Work out the finished part from the listing and answer in its coordinate system (mm). A direction names the side the tool comes from. Coordinates: 2 decimals unless noted, no trailing zeros. Loops run counter-clockwise (first coordinate to the right, second up) from the corner with the lowest first, then second, coordinate; pieces in that order, holes last. Notation, with made-up numbers: M 87,-9.5 L 136,-9.5 A14 ccw 136,4.5 Z; hole C 87,-4.5 d6. An arc over 180 degrees is marked long. Write each question's results on one line, items separated by ' | '.
```python
from build123d import *

# Parameters (mm, degrees)
F0_W     = 2
F0_H     = 35
F1_DEPTH = 22
F2_R     = 1
F3_DEPTH = 25
F4_W     = 1
F4_H     = 35
F4_W_2   = 2
F5_DEPTH = 2
F8_R     = 4.5
F8_R_2   = 2.5
F9_DEPTH = 8.5


# Not quite as in the source:
# - a feature names something its author has since deleted; it is built from what else it names


with BuildPart() as f1:
    # F0 (on Front) → F1 (new body)
    with BuildSketch(Plane.XZ):
        Rectangle(F0_W, F0_H)
    extrude(amount=F1_DEPTH)

    # F2 (on face) → F3 (cut)
    with BuildSketch(Plane(origin=(-1, 0, 0), x_dir=(0, -1, 0), z_dir=(-1, 0, 0))):
        with Locations((5, 10)):
            Circle(F2_R)
        with Locations((15, 10)):
            Circle(F2_R)
        with Locations((15, 0)):
            Circle(F2_R)
        with Locations((5, 0)):
            Circle(F2_R)
        with Locations((5, -10)):
            Circle(F2_R)
        with Locations((15, -10)):
            Circle(F2_R)
    extrude(amount=-F3_DEPTH, mode=Mode.SUBTRACT)

    # F4 (on face) → F5 (join)
    with BuildSketch(Plane.XZ.offset(22)):
        with Locations((-1.5, 0)):
            Rectangle(F4_W, F4_H)
        with Locations((1.5, 0)):
            Rectangle(F4_W, F4_H)
        Rectangle(F4_W_2, F4_H)
    extrude(amount=F5_DEPTH)

    # F8 (on offset) + F6 (on face) → F9 (join)
    with BuildSketch(Plane(origin=(0, 0, 0), x_dir=(1, 0, 0), z_dir=(0, 0, -1))):
        with Locations((0, 26.5)):
            Circle(F8_R)
        with Locations((0, 26.5)):
            Circle(F8_R_2, mode=Mode.SUBTRACT)
    with BuildSketch(Plane(origin=(0, 0, -17.5), x_dir=(1, 0, 0), z_dir=(0, 0, -1))):
        with BuildLine():
            Line((-2, 24), (0, 24))
            Line((0, 24), (2, 24))
            Line((2, 24), (2, 22.4688711259))
            ThreePointArc((2, 22.4688711259), (3.8242646352, 24.1282917549), (4.5, 26.5))
            ThreePointArc((4.5, 26.5), (-2.3717082451, 30.3242646352), (-2, 22.4688711259))
            Line((-2, 22.4688711259), (-2, 24))
        make_face()
        with BuildLine():
            ThreePointArc((0, 24), (-1.767766953, 28.267766953), (2.5, 26.5))
            ThreePointArc((2.5, 26.5), (1.767766953, 24.732233047), (0, 24))
        make_face(mode=Mode.SUBTRACT)
    extrude(amount=-F9_DEPTH)


solid = f1.part
```
1) Find section C-C, the plane y = -15. Give the vertices of the cut face in (x, z).
Check result:
outline: M -1,-17.5 L 1,-17.5 L 1,-11 L -1,-11 Z; M -1,-9 L 1,-9 L 1,-1 L -1,-1 Z; M -1,1 L 1,1 L 1,9 L -1,9 Z; M -1,11 L 1,11 L 1,17.5 L -1,17.5 Z
2) Find section B-B, the plane z = 10. Give the vertices of the cut face in (x, y), and give its area (3 significant figures).
Check result:
outline: M -2,-24 L 2,-24 L 2,-22 L 1,-22 L 1,-16 L -1,-16 L -1,-22 L -2,-22 Z; M -1,-14 L 1,-14 L 1,-6 L -1,-6 Z; M -1,-4 L 1,-4 L 1,0 L -1,0 Z | area: 44.0 mm^2
3) For a pull along X with two mould halves and no side action, classify faces 4 (the face through (0, -29, 4)), 5 (the face through (0, -31, 4)), 6 (the face through (-2, -22.3, 3.6)), 7 (the face through (-2, -29, -9)) as released by +X, released by -X, zero draft, split by the parting line, or undercut.
Check result:
face 4: undercut | face 5: split by the parting line | face 6: released by -X | face 7: zero draft
4) Which of the six approach directions +Z, -Z, +X, -X, +Y, -Y give full straight-line access (tool end or side, diameter ignored) to faces 1 (the face through (-1.5, -22, 0.2)), 2 (the face through (0, -24, -4)), 3 (the face through (0, -24, 13))?
Check result:
face 1: +Z, -Z, -X, +Y | face 2: +X, -X, -Y | face 3: +Z, +X, -X, -Y
5) Given pin 1 Ø2.5 at (x, y) = (1, -28.5) entering from +Z; pin 2 Ø4 at (x, z) = (-2.5, -0.5) entering from -Y; pin 3 Ø5 at (y, z) = (-13.5, -4.5) entering from +X, each flat-ended and moving along its own axis, determine where each tip first touches the part or whether it passes through.
Check result:
pin 1: z = 8.5 | pin 2: y = -30.96 | pin 3: x = 1
6) Find section A-A, the plane z = -10. Give the vertices of the cut face in (x, y), and give its area (3 significant figures).
Check result:
outline: M -2,-22.47 A4.5 ccw long 2,-22.47 L 2,-22 L 1,-22 L 1,-16 L -1,-16 L -1,-22 L -2,-22 Z; M -1,-14 L 1,-14 L 1,-6 L -1,-6 Z; M -1,-4 L 1,-4 L 1,0 L -1,0 Z; hole C 0,-26.5 d5 | area: 80.6 mm^2
7) Straight lines are drawn through the part: probe 1 along Z at (x, y) = (0.25, -5); probe 2 along X at (y, z) = (-26.5, 5.25); probe 3 along Y at (x, z) = (0, 4.25). For each, find the intervals that lie inside material, in ascending order. Write a range as [from, to].
Check result:
probe 1: [-17.5, -11], [-9, -1], [1, 9], [11, 17.5] | probe 2: [-4.5, -2.5], [2.5, 4.5] | probe 3: [-31, -29], [-24, 0]
8) Find section D-D, the plane x = 3. Give the vertices of the cut face in (y, z).
Check result:
outline: M -29.85,-17.5 L -23.15,-17.5 L -23.15,-9 L -29.85,-9 Z; M -29.85,0 L -23.15,0 L -23.15,8.5 L -29.85,8.5 Z
